Autodesk Inventor part; units mm, degrees
ref_plane "YZ Plane" through (0, 0, 0) normal (1, 0, 0) x (0, 1, 0)
ref_plane "XZ Plane" through (0, 0, 0) normal (0, 1, 0) x (-1, 0, 0)
ref_plane "XY Plane" through (0, 0, 0) normal (0, 0, 1) x (1, 0, 0)
sketch "Sketch1" plane through (0, 0, 0) normal (0, 1, 0) x (-1, 0, 0)
  line L0 (304.8, 107.95) -> (-304.8, 107.95)
  line L1 (-304.8, 107.95) -> (-304.8, -107.95)
  line L2 (-304.8, -107.95) -> (304.8, -107.95)
  line L3 (304.8, -107.95) -> (304.8, 107.95)
  line L4 (304.8, 107.95) -> (-304.8, -107.95) construction
  line L5 (-304.8, 107.95) -> (304.8, -107.95) construction
  point P0 (0, 0)
  dimension "length" = 609.6
  dimension "width" = 215.9
extrude "Extrusion1" add sketch "Sketch1" along normal blind 19
sketch "Sketch3" plane through (0, 19, 0) normal (0, 1, 0) x (1, 0, 0)
  line L0 (-304.8, 107.95) -> (-304.8, -107.95)
  line L1 (-304.8, -107.95) -> (304.8, -107.95)
  line L2 (-304.8, -107.95) -> (-285.8, -107.95)
  line L3 (-285.8, -107.95) -> (-285.8, -93.5567)
  line L4 (-285.8, -93.5567) -> (-304.8, -93.5567)
  line L5 (-304.8, -93.5567) -> (-304.8, -107.95)
  point P0 (0, 0)
  dimension "d21" = 19
  dimension "d22" = 14.3933
extrude "Extrusion3" cut sketch "Sketch3" against normal through all
mirror "Mirror2" about plane through (0, 0, 0) normal (0, 0, 1) of "Extrusion3"
sketch "Sketch4" plane through (0, 19, 0) normal (0, 1, 0) x (1, 0, 0)
  line L0 (-304.8, 93.5567) -> (-304.8, -93.5567)
  line L1 (-304.8, -79.1633) -> (-285.8, -79.1633)
  line L2 (-285.8, -79.1633) -> (-285.8, -64.77)
  line L3 (-285.8, -64.77) -> (-304.8, -64.77)
  line L4 (-304.8, -64.77) -> (-304.8, -79.1633)
  line L5 (-304.8, -93.5567) -> (-285.8, -93.5567)
  point P0 (0, 0)
  dimension "d25" = 19
  dimension "d26" = 14.3933
  dimension "d27" = 14.3933
extrude "Extrusion4" cut sketch "Sketch4" against normal through all
pattern_linear "Rectangular Pattern1" count 6 spacing 28.7867 along (0, 0, -1) of "Extrusion4"
mirror "Mirror3" about plane through (0, 0, 0) normal (1, 0, 0) of "Extrusion3", "Mirror2", "Extrusion4", "Rectangular Pattern1"
sketch "Sketch5" plane through (0, 0, 0) normal (0, -1, 0) x (1, 0, 0)
  line L0 (152.4, 57.15) -> (-152.4, 57.15) construction
  line L1 (152.4, 76.2) -> (-152.4, 76.2)
  line L2 (-152.4, 38.1) -> (152.4, 38.1)
  arc A0 (152.4, 38.1) -> (152.4, 76.2) centre (152.4, 57.15) ccw
  arc A1 (-152.4, 76.2) -> (-152.4, 38.1) centre (-152.4, 57.15) ccw
  line L3 (-285.8, 107.95) -> (285.8, 107.95)
  point P0 (0, 0)
  point P1 (0, 57.15)
  dimension "d33" = 38.1
  dimension "d34" = 304.8
  dimension "d35" = 0
  dimension "d36" = 50.8
extrude "Extrusion5" cut sketch "Sketch5" against normal blind 19
equation "\"d21\" = thickness"
equation "\"d25\" = thickness"
equation "\"d37\" = thickness"
properties part number "cabinet-bottom" material "Wood (Birch)"
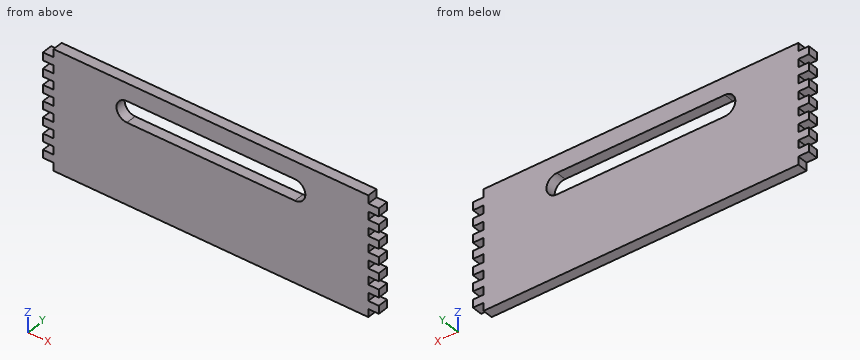
The model under review builds one solid part; all positions refer to its coordinate system, in mm. Coordinates: 2 decimals unless noted, no trailing zeros. Order: outer loops, then holes, each group sorted by start corner. A loop starts at its lowest first (then second) coordinate and runs counter-clockwise, first axis right, second up. Notation, with made-up numbers: M -7.5,11 L 1.5,11 A23 ccw 1.5,41 Z; hole C 49.25,18.5 d10. An arc over 180 degrees is marked long. One line per question, with ' | ' between items.
(1) Add section B-B, the plane x = -33. Write out the cut boundary in (y, z), then the cut area to 3 significant figures.
Geometry results:
outline: M 0,-107.95 L 19,-107.95 L 19,38.1 L 0,38.1 Z; M 0,76.2 L 19,76.2 L 19,107.95 L 0,107.95 Z | area: 3,380 mm²
(2) Add section C-C, the plane z = 13.5. Write out the cut boundary in (x, y).
Geometry results:
outline: M -285.8,0 L 285.8,0 L 285.8,19 L -285.8,19 Z
(3) For probe 1 along Z at (x, y) = (119, 4.5); probe 2 along X at (y, z) = (7.25, 46); probe 3 along Z at (x, y) = (154.5, 8.25), list the stretches that pass through material, from the lowest coordinate up. Write a range as from..to.
Geometry results:
probe 1: z = -107.95..38.1, 76.2..107.95 | probe 2: x = -285.8..-167.85, 167.85..285.8 | probe 3: z = -107.95..38.22, 76.08..107.95
(4) Add section A-A, the plane z = 57.15. Write out the cut boundary in (x, y).
Geometry results:
outline: M -304.8,0 L -171.45,0 L -171.45,19 L -304.8,19 Z; M 171.45,0 L 304.8,0 L 304.8,19 L 171.45,19 Z
(5) Insertion check: pin 1 (5.5 mm diameter, centred on x = -291, y = 8.5, fed in from +Z); pin 2 (10 mm diameter, centred on y = 9.5, z = 13.5, fed in from +X); pin 3 (5.5 mm diameter, centred on x = 299.5, y = 5, fed in from -Z). Each pin has a flat end and moves straight along its axis. Give the tip position at first contact, or say it passes through.
Geometry results:
pin 1: stops at z = 93.56 | pin 2: stops at x = 285.8 | pin 3: stops at z = -93.56
